```python
from build123d import *

# Parameters (mm, degrees)
VENT_EDGE_BREAK_SIZE = 0.127


with BuildPart() as part:
    # Sketch2 → Revolve1 (revolve)
    with BuildSketch(Plane.XY, mode=Mode.PRIVATE) as revolve1_sk:
        Polygon((3.6322, 4.5085), (3.6322, 3.175), (1.27, 3.175), (1.27, 4.5085), (0, 4.5085), (0, 0), (10.4394, 0), (10.4394, 4.5085), (9.1694, 4.5085), (9.1694, 3.175), (6.8072, 3.175), (6.8072, 4.5085), align=None)
    revolve(revolve1_sk.sketch.rotate(Axis((-1.617419624, 0, 0), (1, 0, 0)), 90), axis=Axis((-1.617419624, 0, 0), (1, 0, 0)))

    # vent-edge-break
    vent_edge_break_edges = [part.edges().sort_by_distance(p)[0] for p in [
        (3.6322, 0, -4.5085),
        (6.8072, 0, -4.5085),
        (9.1694, 0, -4.5085),
        (10.4394, 0, -4.5085),
        (0, 0, -4.5085),
        (1.27, 0, -4.5085),
    ]]
    chamfer(vent_edge_break_edges, length=VENT_EDGE_BREAK_SIZE)


solid = part.part
```
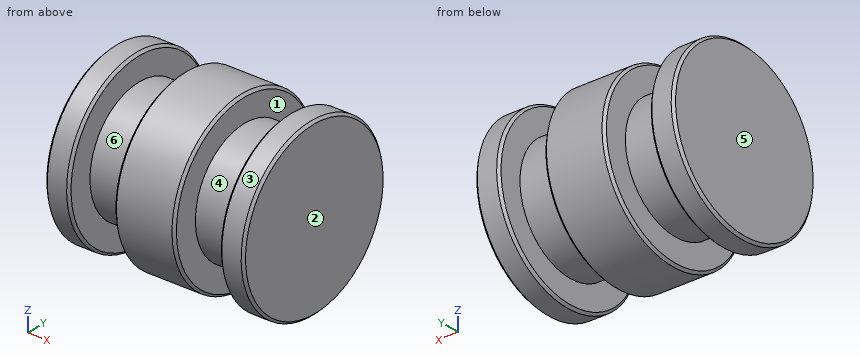
Read the model definition and answer for the solid it produces. Units are mm, in the model's axes. Face numbers are marked on the shaded views. A direction names the side the tool comes from. Give positions to 0.01 mm unless a question says otherwise; leave off trailing zeros. Order: outer loops, then holes, each group sorted by start corner. A loop starts at its lowest first (then second) coordinate and runs counter-clockwise, first axis right, second up.
(1) For the marked faces 1 and 2, determine the directions among +Z, -Z, +X, -X, +Y, -Y from which every point of the face is accessible in a straight line to the end or side of a thin tool.
(2) Given pin 1 (1 mm diameter, centred on x = 8, z = -1, fed in from +Y); pin 2 (2 mm diameter, centred on x = 9, y = 2, fed in from -Z), each flat-ended and moving along its own axis, determine where each tip first touches the part or whether it passes through.
(3) Straight lines are drawn through the part: L1, parallel to X at y = -2.75, z = 2.75; L2, parallel to Z at x = 9.5, y = 2; L3, parallel to Z at x = 8.75, y = 0.5. For each, find the intervals that lie inside material, in ascending order.
(4) For a pull along X with two mould halves and no side action, classify the marked faces 3, 4, 5 and 6 as released by +X, released by -X, zero draft, split by the parting line, or undercut.
(5) Find section C-C (x = 6.5). Give the vertices of the cut face in (y, z).
(6) Find section D-D (x = 9). Give the vertices of the cut face in (y, z) (3 decimals).
Result sheet:
1. face 1: none
1. face 2: +Z, -Z, +X, +Y, -Y
2. pin 1: stops at y = 3.14
2. pin 2: stops at z = -4.39
3. L1: x = 0 to 1.27, 3.63 to 6.81, 9.17 to 10.44
3. L2: z = -4.04 to 4.04
3. L3: z = -3.14 to 3.14
4. face 3: zero draft
4. face 4: undercut
4. face 5: released by -X
4. face 6: undercut
5. outline: circle Ø9.02 at (0, 0)
6. outline: circle Ø6.35 at (0, 0)
